Read the model definition and answer for the solid it produces. Units are mm, in the model's axes. A direction names the side the tool comes from. Give positions to 0.01 mm unless a question says otherwise; leave off trailing zeros. Order: outer loops, then holes, each group sorted by start corner. A loop starts at its lowest first (then second) coordinate and runs counter-clockwise, first axis right, second up. Notation, with made-up numbers: (30.5, -20) - (41.5, -20) arc R23 cw to (41.5, -9) - close; hole circle Ø1 at (-15.5, 15.5). An arc over 180 degrees is marked (long way). Use a Markdown table: item, result. Add a question column.
1. Flat-ended cylindrical pins translate along their axes: P1, Ø6.5, axis at x = 7, y = 189.5, coming from the +Z side; P2, Ø23, axis at x = 47, z = -181, coming from the +Y side; P3, Ø12, axis at x = 26, z = -140, coming from the +Y side. Find the tip coordinate at first contact, or state that the pin passes through.
2. Which of the six approach directions +Z, -Z, +X, -X, +Y, -Y give full straight-line access (tool end or side, diameter ignored) to faces 4 (the flat face through (6, 177.8, -53)), 5 (the flat face through (12.7, 112, -125)), 6 (the flat face through (9, 56, 0)), 7 (the flat face through (6, 203.2, -127)), 8 (the flat face through (6, 191, -146.05))?
3. For a pull along Z with two mould halves and no side action, classify faces 1 (the cylindrical face through (59.685, 6.261, -64.086)), 2 (the flat face through (9, 56, -254)), 3 (the flat face through (101.6, 6, -125)) as released by +Z, released by -Z, zero draft, split by the parting line, or undercut.
4. A cutting plane is placed at C-C on z = -49. Determine the outline of the cut face in (x, y), and give its area (3 significant figures).
5. A cutting plane is placed at D-D on x = 9. Determine the outline of the cut face in (y, z).
6. A cutting plane is placed at B-B on x = 54. Determine the outline of the cut face in (y, z), and give its area (3 significant figures).
7. Consider L1, parallel to Z at x = 63.5, y = 3.5; L2, parallel to Y at x = 75, z = -40. Determine where each line is inside the solid, lowest interval first.
8. A cutting plane is placed at A-A on z = -177.8. Determine the outline of the cut face in (x, y).
Autodesk Inventor part; units mm, degrees
ref_plane "YZ Plane" through (0, 0, 0) normal (1, 0, 0) x (0, 1, 0)
ref_plane "XZ Plane" through (0, 0, 0) normal (0, 1, 0) x (-1, 0, 0)
ref_plane "XY Plane" through (0, 0, 0) normal (0, 0, 1) x (1, 0, 0)
sketch "Sketch1" plane through (0, 0, 0) normal (0, 0, 1) x (1, 0, 0)
  line L0 (0, 232.5603) -> (0, -22.9879)
  line L1 (-15.3679, 0) -> (133.5003, 0)
  line L2 (0, 177.8) -> (0, 22.86)
  line L3 (22.86, 0) -> (101.6, 0)
  line L4 (101.6, 0) -> (101.6, 12.7)
  line L5 (101.6, 12.7) -> (24.13, 12.7)
  line L6 (12.7, 24.13) -> (12.7, 177.8)
  line L7 (12.7, 177.8) -> (0, 177.8)
  arc A0 (0, 22.86) -> (22.86, 0) centre (22.86, 22.86) ccw
  arc A1 (12.7, 24.13) -> (24.13, 12.7) centre (24.13, 24.13) ccw
  dimension "d0" = 22.86
  dimension "d1" = 12.7
  dimension "d2" = 177.8
  dimension "d4" = 12.7
  dimension "d6" = 101.6
  dimension "d7" = 11.43
extrude "Extrusion1" add sketch "Sketch1" against normal blind 254 contours L7 L6 A1 L5 L4 L1 A0 L0
sketch "Sketch2" plane through (24.13, 12.7, 0) normal (0, 1, 0) x (1, 0, 0)
  line L0 (77.47, 0) -> (0, 0)
  line L1 (77.47, 0) -> (77.47, 254)
  point P0 (39.37, 76.2)
  dimension "d10" = 38.1
  dimension "d11" = 76.2
hole "Hole1" at (63.5, 12.7, -76.2) direction (0, -1, 0) diameter 25.4 end through all
pattern_linear "Rectangular Pattern1" count 2 spacing 101.6 along (0, 0, -1) of "Hole1"
sketch "Sketch3" plane through (12.7, 24.13, 0) normal (1, 0, 0) x (0, 0, -1)
  line L0 (0, 153.67) -> (254, 153.67)
  line L1 (0, 0) -> (0, 153.67)
  line L2 (0, 0) -> (254, 0)
  line L3 (107.95, 153.67) -> (107.95, 179.07)
  line L4 (107.95, 179.07) -> (146.05, 179.07)
  line L5 (146.05, 179.07) -> (146.05, 153.67)
  dimension "d22" = 25.4
  dimension "d23" = 38.1
  dimension "d24" = 107.95
extrude "Extrusion2" add sketch "Sketch3" against normal blind 12.7
properties part number "XBRACKET"
Output values:
| question | item | result |
|---|---|---|
| 1 | P1 | z = -107.95 |
| 1 | P2 | y = 12.7 |
| 1 | P3 | y = 13.47 |
| 2 | face 4 | +Z, +X, -X, +Y |
| 2 | face 5 | +Z, -Z, +X, +Y |
| 2 | face 6 | +Z, +X, -X, +Y, -Y |
| 2 | face 7 | +Z, -Z, +X, -X, +Y |
| 2 | face 8 | -Z, +X, -X, +Y |
| 3 | face 1 | undercut |
| 3 | face 2 | released by -Z |
| 3 | face 3 | zero draft |
| 4 | outline | (0, 22.86) arc R22.86 ccw to (22.86, 0) - (101.6, 0) - (101.6, 12.7) - (24.13, 12.7) arc R11.43 cw to (12.7, 24.13) - (12.7, 177.8) - (0, 177.8) - close |
| 4 | area | 3,300 mm² |
| 5 | outline | (4.68, -254) - (177.8, -254) - (177.8, -146.05) - (203.2, -146.05) - (203.2, -107.95) - (177.8, -107.95) - (177.8, 0) - (4.68, 0) - close |
| 6 | outline | (0, -254) - (12.7, -254) - (12.7, -186.23) - (0, -186.23) - close; (0, -169.37) - (12.7, -169.37) - (12.7, -84.63) - (0, -84.63) - close; (0, -67.77) - (12.7, -67.77) - (12.7, 0) - (0, 0) - close |
| 6 | area | 2,800 mm² |
| 7 | L1 | -254 to -190.5, -165.1 to -88.9, -63.5 to 0 |
| 7 | L2 | 0 to 12.7 |
| 8 | outline | (0, 22.86) arc R22.86 ccw to (22.86, 0) - (50.8, 0) - (50.8, 12.7) - (24.13, 12.7) arc R11.43 cw to (12.7, 24.13) - (12.7, 177.8) - (0, 177.8) - close; (76.2, 0) - (101.6, 0) - (101.6, 12.7) - (76.2, 12.7) - close |
